```python
from build123d import *

# Parameters (mm, degrees)
SKETCH1_R           = 12.5
SKETCH1_R_2         = 10
BOSS_EXTRUDE1_DEPTH = 1.5
SKETCH2_R           = 12.5
BOSS_EXTRUDE2_DEPTH = 1.5
SKETCH3_R           = 2.6
CUT_EXTRUDE1_DEPTH  = 2


with BuildPart() as part:
    # Sketch1 → Boss-Extrude1 (new body)
    with BuildSketch(Plane(origin=(0, 0, 0), x_dir=(1, 0, 0), z_dir=(0, 1, 0))):
        with Locations(Location((0, 0, 0), (0, 0, 270))):
            Circle(SKETCH1_R)
        with Locations(Location((0, 0, 0), (0, 0, 270))):
            Circle(SKETCH1_R_2, mode=Mode.SUBTRACT)
    extrude(amount=BOSS_EXTRUDE1_DEPTH)

    # Sketch2 → Boss-Extrude2 (add)
    with BuildSketch(Plane(origin=(0, 1.5, 0), x_dir=(1, 0, 0), z_dir=(0, 1, 0))):
        with Locations(Location((0, 0, 0), (0, 0, 270))):
            Circle(SKETCH2_R)
    extrude(amount=BOSS_EXTRUDE2_DEPTH)

    # Sketch3 → Cut-Extrude1 (cut)
    with BuildSketch(Plane(origin=(0, 3, 0), x_dir=(1, 0, 0), z_dir=(0, 1, 0))):
        with Locations(Location((0, 0, 0), (0, 0, 270))):
            Circle(SKETCH3_R)
    extrude(amount=-CUT_EXTRUDE1_DEPTH, mode=Mode.SUBTRACT)


solid = part.part
```
Read the model definition and answer for the solid it produces. Units are mm, in the model's axes. A direction names the side the tool comes from. Give positions to 0.01 mm unless a question says otherwise; leave off trailing zeros. Write each loop counter-clockwise with the first axis right and the second up, starting at its lowest first coordinate (ties: lowest second). Pieces come first, ordered by that corner, then holes. Notation, with made-up numbers: (32, 1) -> (44, 1) arc R17 ccw to (44, 5) -> close; hole circle Ø6 at (-34.5, -3). An arc over 180 degrees is marked (long way). Answer as a JSON object with one key per item and string values.
1) Section D-D on z = 4.5 is taken. Write down the section's boundary in (x, y), then the cut area to 3 significant figures.
Findings below:
{"outline": "(-11.66, 0) -> (-8.93, 0) -> (-8.93, 1.5) -> (8.93, 1.5) -> (8.93, 0) -> (11.66, 0) -> (11.66, 3) -> (-11.66, 3) -> close", "area": "43.2 mm^2"}
2) Straight lines are drawn through the part: probe 1 along X at (y, z) = (0.1, 0.25); probe 2 along X at (y, z) = (2.35, 0); probe 3 along Y at (x, z) = (3.5, 6.25). For each, find the intervals that lie inside material, in ascending order. Write a range as from..to.
Findings below:
{"probe 1": "x = -12.5..-10, 10..12.5", "probe 2": "x = -12.5..-2.6, 2.6..12.5", "probe 3": "y = 1.5..3"}
3) Section A-A on z = 0 is taken. Write down the section's boundary in (x, y).
Findings below:
{"outline": "(-12.5, 0) -> (-10, 0) -> (-10, 1.5) -> (-2.6, 1.5) -> (-2.6, 3) -> (-12.5, 3) -> close; (2.6, 1.5) -> (10, 1.5) -> (10, 0) -> (12.5, 0) -> (12.5, 3) -> (2.6, 3) -> close"}
4) Section B-B on x = 0 is taken. Write down the section's boundary in (y, z), then the cut area to 3 significant figures.
Findings below:
{"outline": "(0, -12.5) -> (3, -12.5) -> (3, -2.6) -> (1.5, -2.6) -> (1.5, -10) -> (0, -10) -> close; (0, 10) -> (1.5, 10) -> (1.5, 2.6) -> (3, 2.6) -> (3, 12.5) -> (0, 12.5) -> close", "area": "37.2 mm^2"}
5) For a pull along X with two mould halves and no side action, classify faces 1 (the cylindrical face through (0.78, 2.26, 2.48)), 2 (the flat face through (-3, 3, 0)), 3 (the cylindrical face through (3.755, 1.479, 11.923)), 4 (the cylindrical face through (-9.76, 0.74, -2.17)) as pulls with the +X half, pulls with the -X half, needs draft (parallel to the pull), parting line crosses it, or undercut.
Findings below:
{"face 1": "undercut", "face 2": "needs draft", "face 3": "parting line crosses it", "face 4": "undercut"}
6) A tool of negligible diameter and unlimited length cuts with its end or side. For faces 5 (the flat face through (-2, 1.5, 2)), 6 (the flat face through (10.2, 0, -0.1)), from which of +Z, -Z, +X, -X, +Y, -Y can it reach the whole face along a straight path? Write none if from no direction.
Findings below:
{"face 5": "-Y", "face 6": "+Z, -Z, +X, -X, -Y"}
7) Section C-C on y = 0.95 is taken. Write down the section's boundary in (x, z), then the cut area to 3 significant figures.
Findings below:
{"outline": "circle Ø25 at (0, 0); hole circle Ø20 at (0, 0)", "area": "177 mm^2"}
8) A flat-ended cylindrical pin translates along its axis: pin 1 Ø1 at (y, z) = (2, -6.5) entering from +X. Find the tip coordinate at first contact, or state that the pin passes through.
Findings below:
{"pin 1": "stops at x = 10.97"}
